```python
from build123d import *

# Parameters (mm, degrees)
SKETCH1_W           = 25
SKETCH1_H           = 34
SKETCH1_W_2         = 20.5
SKETCH1_H_2         = 20.5
BOSS_EXTRUDE1_DEPTH = 40
SKETCH2_W           = 25
SKETCH2_H           = 34
BOSS_EXTRUDE2_DEPTH = 55
SKETCH3_W           = 25
SKETCH3_H           = 12
BOSS_EXTRUDE3_DEPTH = 20
SKETCH4_W           = 25
SKETCH4_H           = 12
BOSS_EXTRUDE4_DEPTH = 10
SKETCH6_R           = 8
CUT_EXTRUDE1_DEPTH  = 12
FILLET1_R           = 12
SKETCH7_W           = 5.2
SKETCH7_H           = 20.2
CUT_EXTRUDE2_DEPTH  = 28


with BuildPart() as part:
    # Sketch1 → Boss-Extrude1 (new body)
    with BuildSketch(Plane(origin=(0, 0, 0), x_dir=(1, 0, 0), z_dir=(0, 1, 0))):
        with Locations((0, 4.5)):
            Rectangle(SKETCH1_W, SKETCH1_H)
        Rectangle(SKETCH1_W_2, SKETCH1_H_2, mode=Mode.SUBTRACT)
    extrude(amount=BOSS_EXTRUDE1_DEPTH)

    # Sketch2 → Boss-Extrude2 (add)
    with BuildSketch(Plane(origin=(0, 40, 0), x_dir=(1, 0, 0), z_dir=(0, 1, 0))):
        with Locations((0, 4.5)):
            Rectangle(SKETCH2_W, SKETCH2_H)
    extrude(amount=BOSS_EXTRUDE2_DEPTH)

    # Sketch3 → Boss-Extrude3 (add)
    with BuildSketch(Plane(origin=(0, 95, 0), x_dir=(1, 0, 0), z_dir=(0, 1, 0))):
        with Locations((0, 15.5)):
            Rectangle(SKETCH3_W, SKETCH3_H)
    extrude(amount=BOSS_EXTRUDE3_DEPTH)

    # Sketch4 → Boss-Extrude4 (add)
    with BuildSketch(Plane(origin=(0, 115, 0), x_dir=(1, 0, 0), z_dir=(0, 1, 0))):
        with Locations((0, 15.5)):
            Rectangle(SKETCH4_W, SKETCH4_H)
    extrude(amount=BOSS_EXTRUDE4_DEPTH)

    # Sketch6 → Cut-Extrude1 (cut)
    with BuildSketch(Plane.XY.offset(-9.5)):
        with Locations((0, 113)):
            Circle(SKETCH6_R)
    extrude(amount=-CUT_EXTRUDE1_DEPTH, mode=Mode.SUBTRACT)

    # Fillet1
    fillet1_edges = [part.edges().sort_by_distance(p)[0] for p in [
        (-12.5, 125, -15.5),
        (12.5, 125, -15.5),
    ]]
    fillet(fillet1_edges, radius=FILLET1_R)

    # Sketch7 → Cut-Extrude2 (cut)
    with BuildSketch(Plane.XY.offset(12.5)):
        with Locations((-9.9, 80.1)):
            Rectangle(SKETCH7_W, SKETCH7_H)
        with Locations((9.9, 80.1)):
            Rectangle(SKETCH7_W, SKETCH7_H)
    extrude(amount=-CUT_EXTRUDE2_DEPTH, mode=Mode.SUBTRACT)


solid = part.part
```
The model under review builds one solid part; all positions refer to its coordinate system, in mm. A direction names the side the tool comes from. Round coordinates to 2 decimals unless told otherwise and drop trailing zeros. Loops run counter-clockwise (first coordinate to the right, second up) from the corner with the lowest first, then second, coordinate; pieces in that order, holes last. Notation, with made-up numbers: (50, 4.25) -> (92, 4.25) arc R19 ccw to (92, 18.25) -> close; hole circle Ø1 at (79.5, -22). An arc over 180 degrees is marked (long way). Answer as a JSON object with one key per item and string values. Group by question number.
1) For pin 1 Ø1.6 at (x, z) = (-11, 3.5) entering from +Y; pin 2 Ø1.6 at (x, y) = (-8.5, 76.5) entering from +Z; pin 3 Ø10 at (x, z) = (-1.5, 0) entering from -Y, all flat-tipped, find the tip position at first contact; note any pin that passes through.
2) For faces 5 (the face through (-10, 80, -15.5)), 6 (the face through (10, 70, -1)), 7 (the face through (0, 47, 12.5)), 8 (the face through (10.25, 20, 0)), list the 3-axis set-ups (+Z, -Z, +X, -X, +Y, -Y) from which the entire face can be reached by the end or side of a thin tool; tool diameter is ignored.
3) Mouldability with a two-part tool opening along Z and no side actions: class faces 1 (the face through (-10, 70, -1)), 2 (the face through (0, 103, -9.5)), 3 (the face through (0, 62, -21.5)), 4 (the face through (0, 20, 10.25)) as released by +Z, released by -Z, zero draft, split by the parting line, or undercut.
4) We need section B-B on x = -3.75. Write out the cut boundary in (y, z), then the cut area to 3 significant figures.
5) We need section D-D on z = -7.5. Write out the cut boundary in (x, y).
6) We need section C-C on y = 109. Write out the cut boundary in (x, z), then the cut area to 3 significant figures.
7) We need section A-A on y = 16. Write out the cut boundary in (x, z), then the cut area to 3 significant figures.
8) For line 1 (Z direction, x = 9.75, y = 39); line 2 (Y direction, x = 0, z = -13); line 3 (X direction, y = 35, z = -3), list the stretches that pass through material, from the lowest coordinate up. Write a range as [from, to].
Result set:
{
 "1": {"pin 1": "y = 95", "pin 2": "z = -15.5", "pin 3": "y = 40"},
 "2": {"face 5": "+Z, -X", "face 6": "+Z, +X", "face 7": "+Z, +X, -X, +Y, -Y", "face 8": "-Y"},
 "3": {"face 1": "zero draft", "face 2": "released by +Z", "face 3": "released by -Z", "face 4": "undercut"},
 "4": {"outline": "(0, -21.5) -> (105.93, -21.5) -> (105.93, -9.5) -> (95, -9.5) -> (95, 12.5) -> (0, 12.5) -> (0, 10.25) -> (40, 10.25) -> (40, -10.25) -> (0, -10.25) -> close; (120.07, -21.5) -> (124.55, -21.5) -> (124.55, -9.5) -> (120.07, -9.5) -> close", "area": "2,600 mm²"},
 "5": {"outline": "(-12.5, 0) -> (-10.25, 0) -> (-10.25, 40) -> (10.25, 40) -> (10.25, 0) -> (12.5, 0) -> (12.5, 70) -> (7.3, 70) -> (7.3, 90.2) -> (12.5, 90.2) -> (12.5, 95) -> (-12.5, 95) -> (-12.5, 90.2) -> (-7.3, 90.2) -> (-7.3, 70) -> (-12.5, 70) -> close"},
 "6": {"outline": "(-12.5, -21.5) -> (-6.93, -21.5) -> (-6.93, -9.5) -> (-12.5, -9.5) -> close; (6.93, -21.5) -> (12.5, -21.5) -> (12.5, -9.5) -> (6.93, -9.5) -> close", "area": "134 mm²"},
 "7": {"outline": "(-12.5, -21.5) -> (12.5, -21.5) -> (12.5, 12.5) -> (-12.5, 12.5) -> close; hole (-10.25, -10.25) -> (10.25, -10.25) -> (10.25, 10.25) -> (-10.25, 10.25) -> close", "area": "430 mm²"},
 "8": {"line 1": "[-21.5, -10.25], [10.25, 12.5]", "line 2": "[0, 105], [121, 125]", "line 3": "[-12.5, -10.25], [10.25, 12.5]"}
}
